from build123d import *

# Parameters (mm, degrees)
SKETCH1_W                                        = 50.8
SKETCH1_H                                        = 19.05
SKETCH1_R                                        = 3
BOSS_EXTRUDE1_DEPTH                              = 12.7
CBORE_FOR_M3_HEX_HEAD_MACHINE_SCREW1_D           = 3.4
CBORE_FOR_M3_HEX_HEAD_MACHINE_SCREW1_CBORE_D     = 8.4
CBORE_FOR_M3_HEX_HEAD_MACHINE_SCREW1_CBORE_DEPTH = 2.3


with BuildPart() as part:
    # Sketch1 → Boss-Extrude1 (new body)
    with BuildSketch(Plane.XY):
        Rectangle(SKETCH1_W, SKETCH1_H)
        with Locations((-14.2875, 3.525)):
            Circle(SKETCH1_R, mode=Mode.SUBTRACT)
        with Locations((14.2875, 3.525)):
            Circle(SKETCH1_R, mode=Mode.SUBTRACT)
    extrude(amount=BOSS_EXTRUDE1_DEPTH)

    # CBORE for M3 Hex Head Machine Screw1 (through all)
    with Locations(Plane(origin=(0, 9.525, 0), x_dir=(1, 0, 0), z_dir=(0, 1, 0))):
        with Locations((-20.6375, -6.35), (20.6375, -6.35)):
            CounterBoreHole(CBORE_FOR_M3_HEX_HEAD_MACHINE_SCREW1_D / 2, CBORE_FOR_M3_HEX_HEAD_MACHINE_SCREW1_CBORE_D / 2, CBORE_FOR_M3_HEX_HEAD_MACHINE_SCREW1_CBORE_DEPTH)


solid = part.part
Verification items for the finished model (mm, model axes). A direction names the side the tool comes from. Give positions to 0.01 mm unless a question says otherwise; leave off trailing zeros. Loops run counter-clockwise (first coordinate to the right, second up) from the corner with the lowest first, then second, coordinate; pieces in that order, holes last.
1. Go/stop test with flat-tipped pins: P1, Ø4, axis at x = -20.64, z = 6.35, coming from the +Y side (3 decimals); P2, Ø8, axis at x = 14.29, y = 3.52, coming from the -Z side; P3, Ø2, axis at x = 20.64, z = 6.35, coming from the -Y side. Record where each tip stops, or that it passes through.
Derived:
P1: stops at y = 7.225
P2: stops at z = 0
P3: passes through
2. Cross-section at D-D on y = 8.5. Record the cut outline in (x, z).
Derived:
outline: (-25.4, 0) - (25.4, 0) - (25.4, 12.7) - (-25.4, 12.7) - close; hole circle Ø8.4 at (-20.64, 6.35); hole circle Ø8.4 at (20.64, 6.35)
3. Release check for a two-part mould opening along Y. For faces 1 (the cylindrical face through (19.73, 8.39, 10.45)), 2 (the flat face through (20.6, 7.225, 8.2)), 3 (the cylindrical face through (11.29, 3.66, 6.26)) record: +Y half, -Y half, draft (parallel to the pull), parting line (faces both ways), or undercut.
Derived:
face 1: draft
face 2: +Y half
face 3: undercut
4. Cross-section at B-B on z = 7.5. Record the cut outline in (x, y) (1 decimal), and give its area (3 significant figures).
Derived:
outline: (-25.4, -9.5) - (-21.9, -9.5) - (-21.9, 7.2) - (-24.7, 7.2) - (-24.7, 9.5) - (-25.4, 9.5) - close; (-19.4, -9.5) - (19.4, -9.5) - (19.4, 7.2) - (16.6, 7.2) - (16.6, 9.5) - (-16.6, 9.5) - (-16.6, 7.2) - (-19.4, 7.2) - close; (21.9, -9.5) - (25.4, -9.5) - (25.4, 9.5) - (24.7, 9.5) - (24.7, 7.2) - (21.9, 7.2) - close; hole circle Ø6 at (-14.3, 3.5); hole circle Ø6 at (14.3, 3.5)
area: 790 mm2
5. Tool access check on faces 4 (the cylindrical face through (-22.26, -1.27, 5.84)), 5 (the flat face through (-20.7, 7.225, 8.2)). Record the directions out of +Z, -Z, +X, -X, +Y, -Y that give a thin tool (end or side, any length) a straight path to the whole face; none if there is none.
Derived:
face 4: +Y, -Y
face 5: +Y
6. Material ranges on probe 1 along X at (y, z) = (-3.75, 6.35); probe 2 along X at (y, z) = (3.5, 10); probe 3 along Y at (x, z) = (15, 1.5) (3 decimals), recorded low to high.
Derived:
probe 1: x = -25.4 to -22.34, -18.94 to 18.94, 22.34 to 25.4
probe 2: x = -25.4 to -17.29, -11.29 to 11.29, 17.29 to 25.4
probe 3: y = -9.525 to 0.611, 6.439 to 9.525
7. Cross-section at C-C on z = 9.75. Record the cut outline in (x, y) (1 decimal).
Derived:
outline: (-25.4, -9.5) - (25.4, -9.5) - (25.4, 9.5) - (23.1, 9.5) - (23.1, 7.2) - (18.2, 7.2) - (18.2, 9.5) - (-18.2, 9.5) - (-18.2, 7.2) - (-23.1, 7.2) - (-23.1, 9.5) - (-25.4, 9.5) - close; hole circle Ø6 at (-14.3, 3.5); hole circle Ø6 at (14.3, 3.5)
8. Cross-section at A-A on y = -4. Record the cut outline in (x, z).
Derived:
outline: (-25.4, 0) - (25.4, 0) - (25.4, 12.7) - (-25.4, 12.7) - close; hole circle Ø3.4 at (-20.64, 6.35); hole circle Ø3.4 at (20.64, 6.35)
